The listing builds one solid part. Answer for the finished solid, in the listing's coordinates (mm). A direction names the side the tool comes from. Give positions to 0.01 mm unless a question says otherwise; leave off trailing zeros. Order: outer loops, then holes, each group sorted by start corner. A loop starts at its lowest first (then second) coordinate and runs counter-clockwise, first axis right, second up. Notation, with made-up numbers: (-27, -8) -> (25, -8) arc R33 cw to (25, 30) -> close; hole circle Ø1 at (21, 45.5). An arc over 180 degrees is marked (long way). Write item = value, one per line. Start each with the question number.
```python
from build123d import *


with BuildPart() as part:
    # 草图1 → 旋转1 (revolve)
    with BuildSketch(Plane.XY, mode=Mode.PRIVATE) as revolve_1_sk:
        with BuildLine():
            Line((0, 0), (5.8, 0))
            Line((5.8, 0), (5.8, 7.4))
            Line((5.8, 7.4), (6.8, 7.4))
            Line((6.8, 7.4), (6.8, 10.75))
            Line((6.8, 10.75), (8.5, 10.75))
            Line((8.5, 10.75), (8.5, 16.4))
            Line((8.5, 16.4), (7.984359711, 16.4))
            ThreePointArc((7.984359711, 16.4), (4.183300133, 18.260389216), (0, 18.9))
            Line((0, 18.9), (0, 0))
        make_face()
    revolve(revolve_1_sk.sketch.rotate(Axis((0, 18.9, 0), (0, -1, 0)), 90), axis=Axis((0, 18.9, 0), (0, -1, 0)))


solid = part.part
```
Item 1: A cutting plane is placed at C-C, the plane y = 8.25. Write down the section's boundary in (x, z).
Item 2: Consider L1, parallel to Z at x = 0.25, y = 14.5; L2, parallel to X at y = 5.5, z = 0.25. Determine where each line is inside the solid, lowest interval first. Write a range as from..to.
Item 3: A cutting plane is placed at A-A, the plane z = 0. Write down the section's boundary in (x, y), plus the area to 3 significant figures.
Item 4: A cutting plane is placed at D-D, the plane z = 4.25. Write down the section's boundary in (x, y).
Item 5: A cutting plane is placed at B-B, the plane x = 0. Write down the section's boundary in (y, z), plus the area to 3 significant figures.
Item 6: Which of the six approach directions +Z, -Z, +X, -X, +Y, -Y give full straight-line access (tool end or side, diameter ignored) to faces 1 (the flat face through (2, 16.4, -8)), 2 (the flat face through (0, 0, 0)), 3 (the cylindrical face through (-0.255, 3.752, -5.794))?
Item 7: Flat-ended cylindrical pins translate along their axes: pin 1 (1.5 mm diameter, centred on x = -5, y = 5.5, fed in from -Z); pin 2 (4 mm diameter, centred on y = 4, z = 3.5, fed in from -X); pin 3 (4 mm diameter, centred on x = 3, z = 2.5, fed in from +Y). Find the tip coordinate at first contact, or state that the pin passes through.
Check values:
q1.outline = circle Ø13.6 at (0, 0)
q2.L1 = -8.5..8.5
q2.L2 = -5.79..5.79
q3.outline = (-8.5, 10.75) -> (-6.8, 10.75) -> (-6.8, 7.4) -> (-5.8, 7.4) -> (-5.8, 0) -> (5.8, 0) -> (5.8, 7.4) -> (6.8, 7.4) -> (6.8, 10.75) -> (8.5, 10.75) -> (8.5, 16.4) -> (7.98, 16.4) arc R14 ccw to (-7.98, 16.4) -> (-8.5, 16.4) -> close
q3.area = 255 mm^2
q4.outline = (-7.36, 10.75) -> (-5.31, 10.75) -> (-5.31, 7.4) -> (-3.95, 7.4) -> (-3.95, 0) -> (3.95, 0) -> (3.95, 7.4) -> (5.31, 7.4) -> (5.31, 10.75) -> (7.36, 10.75) -> (7.36, 16.4) -> (6.76, 16.4) arc R13.34 ccw to (-6.76, 16.4) -> (-7.36, 16.4) -> close
q5.outline = (0, -5.8) -> (7.4, -5.8) -> (7.4, -6.8) -> (10.75, -6.8) -> (10.75, -8.5) -> (16.4, -8.5) -> (16.4, -7.98) arc R14 ccw to (16.4, 7.98) -> (16.4, 8.5) -> (10.75, 8.5) -> (10.75, 6.8) -> (7.4, 6.8) -> (7.4, 5.8) -> (0, 5.8) -> close
q5.area = 255 mm^2
q6.face_1 = +Y
q6.face_2 = +Z, -Z, +X, -X, -Y
q6.face_3 = -Y
q7.pin_1 = -3.95
q7.pin_2 = -5.6
q7.pin_3 = 18.77
